Verification items for the finished model (mm, model axes). A direction names the side the tool comes from. Coordinates: 2 decimals unless noted, no trailing zeros. Order: outer loops, then holes, each group sorted by start corner. A loop starts at its lowest first (then second) coordinate and runs counter-clockwise, first axis right, second up. Notation, with made-up numbers: (30, -9.5) -> (44, -9.5) arc R28 cw to (44, 19.5) -> close; hole circle Ø7 at (-16.5, -39.5). An arc over 180 degrees is marked (long way). Use CSV: the item, a comma, the result in double quotes. Start each with the question number.
1) Scan lines: line 1 along Y through (x, z) = (47.75, 0.7); line 2 along X through (y, z) = (13, 1.4); line 3 along X through (y, z) = (8, 0.85). Record each from-to range of solid material in increasing order.
2) Sectioned sample at A-A on y = 7. Record the boundary of the cut face in (x, z).
3) Go/stop test with a flat-tipped pin: pin 1 (3 mm diameter, centred on x = 47.75, y = 7, fed in from -Z). Record where the tip stops, or that it passes through.
4) Release check for a two-part mould opening along X. For faces 1 (the flat face through (51, 7, 1)), 2 (the flat face through (19, 7, 0)), 3 (the flat face through (24.5, 13, 1)) record: released by +X, released by -X, zero draft, split by the parting line, or undercut.
5) Sectioned sample at C-C on z = 0.9. Record the boundary of the cut face in (x, y).
6) Sectioned sample at B-B on x = 47.75. Record the boundary of the cut face in (y, z), then the cut area to 3 significant figures.
7) Sectioned sample at D-D on y = 11.25. Record the boundary of the cut face in (x, z).
8) Tool access check on faces 4 (the flat face through (12, 14, 1)), 5 (the flat face through (26.5, 13, 1)). Record the directions out of +Z, -Z, +X, -X, +Y, -Y that give a thin tool (end or side, any length) a straight path to the whole face; none if there is none.
from build123d import *

# Parameters (mm, degrees)
SKETCH_W     = 51
SKETCH_H     = 14
PAD_DEPTH    = 2
SKETCH001_R  = 1.25
POCKET_DEPTH = 5


with BuildPart() as part:
    # Sketch → Pad (new body)
    with BuildSketch(Plane.XY):
        with Locations((25.5, 7)):
            Rectangle(SKETCH_W, SKETCH_H)
    extrude(amount=PAD_DEPTH)

    # Sketch001 (on Face6 of Pad) → Pocket (cut)
    with BuildSketch(Plane.XY.offset(2)):
        with Locations((3.25, 7)):
            Circle(SKETCH001_R)
        with Locations((47.75, 7)):
            Circle(SKETCH001_R)
        with BuildLine():
            Line((24.5, 12.408327), (24.5, 14))
            Line((24.5, 14), (26.5, 14))
            Line((26.5, 14), (26.5, 12.408327))
            ThreePointArc((24.5, 12.408327), (25.5, 1.5), (26.5, 12.408327))
        make_face()
    extrude(amount=-POCKET_DEPTH, mode=Mode.SUBTRACT)


solid = part.part
Answers follow:
1,line 1,"y = 0 to 5.75, 8.25 to 14"
1,line 2,"x = 0 to 24.5, 26.5 to 51"
1,line 3,"x = 0 to 2.5, 4 to 20.09, 30.91 to 47, 48.5 to 51"
2,outline,"(0, 0) -> (2, 0) -> (2, 2) -> (0, 2) -> close; (4.5, 0) -> (20, 0) -> (20, 2) -> (4.5, 2) -> close; (31, 0) -> (46.5, 0) -> (46.5, 2) -> (31, 2) -> close; (49, 0) -> (51, 0) -> (51, 2) -> (49, 2) -> close"
3,pin 1,"stops at z = 0"
4,face 1,"released by +X"
4,face 2,"zero draft"
4,face 3,"undercut"
5,outline,"(0, 0) -> (51, 0) -> (51, 14) -> (26.5, 14) -> (26.5, 12.41) arc R5.5 cw (long way) to (24.5, 12.41) -> (24.5, 14) -> (0, 14) -> close; hole circle Ø2.5 at (3.25, 7); hole circle Ø2.5 at (47.75, 7)"
6,outline,"(0, 0) -> (5.75, 0) -> (5.75, 2) -> (0, 2) -> close; (8.25, 0) -> (14, 0) -> (14, 2) -> (8.25, 2) -> close"
6,area,"23.0 mm²"
7,outline,"(0, 0) -> (22.01, 0) -> (22.01, 2) -> (0, 2) -> close; (28.99, 0) -> (51, 0) -> (51, 2) -> (28.99, 2) -> close"
8,face 4,"+Z, -Z, +X, -X, +Y"
8,face 5,"+Z, -Z, +Y"
